```python
from build123d import *

# Parameters (mm, degrees)
F1_DEPTH     = 17.5
F2_T1_DEPTH  = 22.5
F3_T1_DEPTH  = 7
F3_T4_ANGLE  = 168.6544636073
F3_T6_ANGLE  = 168.6544636073
F3_T8_ANGLE  = 180
F3_T10_ANGLE = 168.6544636073
F3_T12_ANGLE = 168.6544636073
F3_T14_ANGLE = 180
F3_T16_ANGLE = 168.6544636073
F3_T18_ANGLE = 168.6544636073
F3_T20_ANGLE = 180
F3_T22_ANGLE = 168.6544636073
F3_T24_ANGLE = 168.6544636073
F3_T26_ANGLE = 180


# Not quite as in the source:
# - a fillet or chamfer that OpenCascade refuses, or shapes differently, is made with other operations: its cross-section is extruded or revolved along the edge and cut away or added


with BuildPart() as f1:
    # F0 (on Top) → F1 (new body)
    with BuildSketch(Plane.XY):
        with BuildLine():
            ThreePointArc((0, -2.75), (-2.75, 0), (0, 2.75))
            Line((0, 2.75), (8, 2.75))
            Line((8, 2.75), (8, 4.25))
            Line((8, 4.25), (0, 4.25))
            ThreePointArc((0, 4.25), (-4.25, 0), (0, -4.25))
            Line((0, -4.25), (8, -4.25))
            Line((8, -4.25), (8, -2.75))
            Line((8, -2.75), (0, -2.75))
        make_face()
    extrude(amount=F1_DEPTH)

    # F2: fillet of radius 1 on 4 edges, made by hand

    # F2_s2 → F2_t1 (cut)
    with BuildSketch(Plane.XY.offset(-2.5)):
        with BuildLine():
            ThreePointArc((8, -3.75), (7.7071067812, -3.0428932188), (7, -2.75))
            Line((7, -2.75), (8, -2.75))
            Line((8, -2.75), (8, -3.75))
        make_face()
        with BuildLine():
            ThreePointArc((7, -4.25), (7.7071067812, -3.9571067812), (8, -3.25))
            Line((8, -3.25), (8, -4.25))
            Line((8, -4.25), (7, -4.25))
        make_face()
        with BuildLine():
            ThreePointArc((7, 2.75), (7.7071067812, 3.0428932188), (8, 3.75))
            Line((8, 3.75), (8, 2.75))
            Line((8, 2.75), (7, 2.75))
        make_face()
        with BuildLine():
            ThreePointArc((8, 3.25), (7.7071067812, 3.9571067812), (7, 4.25))
            Line((7, 4.25), (8, 4.25))
            Line((8, 4.25), (8, 3.25))
        make_face()
    extrude(amount=F2_T1_DEPTH, mode=Mode.SUBTRACT)

    # F3: fillet of radius 0.65 on 20 edges, made by hand

    # F3_s2 → F3_t1 (cut)
    with BuildSketch(Plane.YZ):
        with BuildLine():
            ThreePointArc((-2.75, 0.65), (-2.9403805922, 0.1903805922), (-3.4, 0))
            Line((-3.4, 0), (-2.75, 0))
            Line((-2.75, 0), (-2.75, 0.65))
        make_face()
        with BuildLine():
            ThreePointArc((-3.6, 0), (-4.0596194078, 0.1903805922), (-4.25, 0.65))
            Line((-4.25, 0.65), (-4.25, 0))
            Line((-4.25, 0), (-3.6, 0))
        make_face()
        with BuildLine():
            ThreePointArc((3.6, 0), (4.0596194078, 0.1903805922), (4.25, 0.65))
            Line((4.25, 0.65), (4.25, 0))
            Line((4.25, 0), (3.6, 0))
        make_face()
        with BuildLine():
            ThreePointArc((2.75, 0.65), (2.9403805922, 0.1903805922), (3.4, 0))
            Line((3.4, 0), (2.75, 0))
            Line((2.75, 0), (2.75, 0.65))
        make_face()
        with BuildLine():
            ThreePointArc((-2.75, 16.85), (-2.9403805922, 17.3096194078), (-3.4, 17.5))
            Line((-3.4, 17.5), (-2.75, 17.5))
            Line((-2.75, 17.5), (-2.75, 16.85))
        make_face()
        with BuildLine():
            ThreePointArc((-3.6, 17.5), (-4.0596194078, 17.3096194078), (-4.25, 16.85))
            Line((-4.25, 16.85), (-4.25, 17.5))
            Line((-4.25, 17.5), (-3.6, 17.5))
        make_face()
        with BuildLine():
            ThreePointArc((3.6, 17.5), (4.0596194078, 17.3096194078), (4.25, 16.85))
            Line((4.25, 16.85), (4.25, 17.5))
            Line((4.25, 17.5), (3.6, 17.5))
        make_face()
        with BuildLine():
            ThreePointArc((2.75, 16.85), (2.9403805922, 17.3096194078), (3.4, 17.5))
            Line((3.4, 17.5), (2.75, 17.5))
            Line((2.75, 17.5), (2.75, 16.85))
        make_face()
    extrude(amount=F3_T1_DEPTH, mode=Mode.SUBTRACT)

    # F3_s3 → F3_t4 (revolve, cut)
    with BuildSketch(Plane.YZ.offset(7)):
        with BuildLine():
            ThreePointArc((-3.4, 0), (-2.9403805922, 0.1903805922), (-2.75, 0.65))
            Line((-2.75, 0.65), (-2.75, 0))
            Line((-2.75, 0), (-3.4, 0))
        make_face()
    revolve(axis=Axis((7, -3.75, 0), (0, 0, -1)), revolution_arc=F3_T4_ANGLE, mode=Mode.SUBTRACT)

    # F3_s5 → F3_t6 (revolve, cut)
    with BuildSketch(Plane(origin=(7.3559574547, -1.4759459573, 0), x_dir=(0, 0, 1), z_dir=(-0.9804586187, 0.1967254356, 0))):
        with BuildLine():
            ThreePointArc((0, -1.4594124616), (0.1903805922, -0.9997930538), (0.65, -0.8094124616))
            Line((0.65, -0.8094124616), (0, -0.8094124616))
            Line((0, -0.8094124616), (0, -1.4594124616))
        make_face()
    revolve(axis=Axis((7, -3.25, 0), (0, 0, -1)), revolution_arc=F3_T6_ANGLE, mode=Mode.SUBTRACT)

    # F3_s7 → F3_t8 (revolve, cut)
    with BuildSketch(Plane.YZ):
        with BuildLine():
            ThreePointArc((3.6, 0), (4.0596194078, 0.1903805922), (4.25, 0.65))
            Line((4.25, 0.65), (4.25, 0))
            Line((4.25, 0), (3.6, 0))
        make_face()
    revolve(axis=Axis((0, 0, 0), (0, 0, 1)), revolution_arc=F3_T8_ANGLE, mode=Mode.SUBTRACT)

    # F3_s9 → F3_t10 (revolve, cut)
    with BuildSketch(Plane.YZ.offset(7)):
        with BuildLine():
            ThreePointArc((3.6, 0), (4.0596194078, 0.1903805922), (4.25, 0.65))
            Line((4.25, 0.65), (4.25, 0))
            Line((4.25, 0), (3.6, 0))
        make_face()
    revolve(axis=Axis((7, 3.25, 0), (0, 0, -1)), revolution_arc=F3_T10_ANGLE, mode=Mode.SUBTRACT)

    # F3_s11 → F3_t12 (revolve, cut)
    with BuildSketch(Plane(origin=(6.0057894127, -1.2050396782, 0), x_dir=(0, 0, 1), z_dir=(-0.9804586187, 0.1967254356, 0))):
        with BuildLine():
            ThreePointArc((0, 5.4037978693), (0.1903805922, 5.8634172771), (0.65, 6.0537978693))
            Line((0.65, 6.0537978693), (0, 6.0537978693))
            Line((0, 6.0537978693), (0, 5.4037978693))
        make_face()
    revolve(axis=Axis((7, 3.75, 0), (0, 0, -1)), revolution_arc=F3_T12_ANGLE, mode=Mode.SUBTRACT)

    # F3_s13 → F3_t14 (revolve, cut)
    with BuildSketch(Plane.YZ):
        with BuildLine():
            ThreePointArc((-2.75, 0.65), (-2.9403805922, 0.1903805922), (-3.4, 0))
            Line((-3.4, 0), (-2.75, 0))
            Line((-2.75, 0), (-2.75, 0.65))
        make_face()
    revolve(axis=Axis((0, 0, 0), (0, 0, -1)), revolution_arc=F3_T14_ANGLE, mode=Mode.SUBTRACT)

    # F3_s15 → F3_t16 (revolve, cut)
    with BuildSketch(Plane.YZ.offset(7)):
        with BuildLine():
            ThreePointArc((-3.4, 17.5), (-2.9403805922, 17.3096194078), (-2.75, 16.85))
            Line((-2.75, 16.85), (-2.75, 17.5))
            Line((-2.75, 17.5), (-3.4, 17.5))
        make_face()
    revolve(axis=Axis((7, -3.75, 17.5), (0, 0, -1)), revolution_arc=F3_T16_ANGLE, mode=Mode.SUBTRACT)

    # F3_s17 → F3_t18 (revolve, cut)
    with BuildSketch(Plane(origin=(7.3559574547, -1.4759459573, 0), x_dir=(0, 0, 1), z_dir=(-0.9804586187, 0.1967254356, 0))):
        with BuildLine():
            ThreePointArc((17.5, -1.4594124616), (17.3096194078, -0.9997930538), (16.85, -0.8094124616))
            Line((16.85, -0.8094124616), (17.5, -0.8094124616))
            Line((17.5, -0.8094124616), (17.5, -1.4594124616))
        make_face()
    revolve(axis=Axis((7, -3.25, 17.5), (0, 0, -1)), revolution_arc=F3_T18_ANGLE, mode=Mode.SUBTRACT)

    # F3_s19 → F3_t20 (revolve, cut)
    with BuildSketch(Plane.YZ):
        with BuildLine():
            ThreePointArc((3.6, 17.5), (4.0596194078, 17.3096194078), (4.25, 16.85))
            Line((4.25, 16.85), (4.25, 17.5))
            Line((4.25, 17.5), (3.6, 17.5))
        make_face()
    revolve(axis=Axis((0, 0, 17.5), (0, 0, 1)), revolution_arc=F3_T20_ANGLE, mode=Mode.SUBTRACT)

    # F3_s21 → F3_t22 (revolve, cut)
    with BuildSketch(Plane.YZ.offset(7)):
        with BuildLine():
            ThreePointArc((3.6, 17.5), (4.0596194078, 17.3096194078), (4.25, 16.85))
            Line((4.25, 16.85), (4.25, 17.5))
            Line((4.25, 17.5), (3.6, 17.5))
        make_face()
    revolve(axis=Axis((7, 3.25, 17.5), (0, 0, -1)), revolution_arc=F3_T22_ANGLE, mode=Mode.SUBTRACT)

    # F3_s23 → F3_t24 (revolve, cut)
    with BuildSketch(Plane(origin=(6.0057894127, -1.2050396782, 0), x_dir=(0, 0, 1), z_dir=(-0.9804586187, 0.1967254356, 0))):
        with BuildLine():
            ThreePointArc((17.5, 5.4037978693), (17.3096194078, 5.8634172771), (16.85, 6.0537978693))
            Line((16.85, 6.0537978693), (17.5, 6.0537978693))
            Line((17.5, 6.0537978693), (17.5, 5.4037978693))
        make_face()
    revolve(axis=Axis((7, 3.75, 17.5), (0, 0, -1)), revolution_arc=F3_T24_ANGLE, mode=Mode.SUBTRACT)

    # F3_s25 → F3_t26 (revolve, cut)
    with BuildSketch(Plane.YZ):
        with BuildLine():
            ThreePointArc((-2.75, 16.85), (-2.9403805922, 17.3096194078), (-3.4, 17.5))
            Line((-3.4, 17.5), (-2.75, 17.5))
            Line((-2.75, 17.5), (-2.75, 16.85))
        make_face()
    revolve(axis=Axis((0, 0, 17.5), (0, 0, -1)), revolution_arc=F3_T26_ANGLE, mode=Mode.SUBTRACT)


solid = f1.part
```
Geometry check sheet. Reference: the model listing, model coordinates, mm. A direction names the side the tool comes from. Coordinates: 2 decimals unless noted, no trailing zeros. Loops run counter-clockwise (first coordinate to the right, second up) from the corner with the lowest first, then second, coordinate; pieces in that order, holes last.
Item 1: Sectioned sample at B-B, the plane y = 0. Record the boundary of the cut face in (x, z).
Item 2: Sectioned sample at A-A, the plane x = 6.75. Record the boundary of the cut face in (y, z), then the cut area to 3 significant figures.
Item 3: Go/stop test with flat-tipped pins: pin 1 Ø5 at (y, z) = (0, 11) entering from +X; pin 2 Ø1.5 at (x, z) = (-2, 5) entering from -Y; pin 3 Ø1.5 at (x, z) = (-1, 10.5) entering from +Y; pin 4 Ø2 at (x, y) = (3.5, 1) entering from +Z. Record where each tip stops, or that it passes through.
Item 4: Thickness scan on line 1 (Y direction, x = 5.5, z = 5.75); line 2 (Y direction, x = -1.75, z = 9.5); line 3 (Z direction, x = -2, y = -3.5). Record the ranges inside material, lowest first.
Item 5: Access from +Z, -Z, +X, -X, +Y, -Y to the whole of each face (thin tool, end or side, straight path). Record for faces 1 (the face through (7.62, -2.965, 8.637)), 2 (the face through (7.605, -4.046, 8.637)).
Item 6: Sectioned sample at C-C, the plane z = 2.25. Record the boundary of the cut face in (x, y), then the cut area to 3 significant figures.
Item 7: Release check for a two-part mould opening along Y. For faces 3 (the face through (-2.75, -0.06, 8.64)), 4 (the face through (4, 4.25, 9)), 5 (the face through (3, -4.25, 9)), 6 (the face through (-4.25, 0.09, 8.64)) record: released by +Y, released by -Y, zero draft, split by the parting line, or undercut.
Check result:
1. outline: (-4.25, 0.65) arc R0.65 ccw to (-3.6, 0) - (-3.4, 0) arc R0.65 ccw to (-2.75, 0.65) - (-2.75, 16.85) arc R0.65 ccw to (-3.4, 17.5) - (-3.6, 17.5) arc R0.65 ccw to (-4.25, 16.85) - close
2. outline: (-4.25, 0.65) arc R0.65 ccw to (-3.6, 0) - (-3.4, 0) arc R0.65 ccw to (-2.75, 0.65) - (-2.75, 16.85) arc R0.65 ccw to (-3.4, 17.5) - (-3.6, 17.5) arc R0.65 ccw to (-4.25, 16.85) - close; (2.75, 0.65) arc R0.65 ccw to (3.4, 0) - (3.6, 0) arc R0.65 ccw to (4.25, 0.65) - (4.25, 16.85) arc R0.65 ccw to (3.6, 17.5) - (3.4, 17.5) arc R0.65 ccw to (2.75, 16.85) - close
2. area: 51.8 mm2
3. pin 1: stops at x = -1.15
3. pin 2: stops at y = -4.06
3. pin 3: stops at y = 4.24
3. pin 4: passes through
4. line 1: y = -4.25 to -2.75, 2.75 to 4.25
4. line 2: y = -3.87 to -2.12, 2.12 to 3.87
4. line 3: z = 0.16 to 17.34
5. face 1: +Z, -Z, +X
5. face 2: +Z, -Z, +X, -Y
6. outline: (0, -4.25) - (7, -4.25) arc R1 ccw to (7.97, -3.5) arc R1 ccw to (7, -2.75) - (0, -2.75) arc R2.75 cw to (0, 2.75) - (7, 2.75) arc R1 ccw to (7.97, 3.5) arc R1 ccw to (7, 4.25) - (0, 4.25) arc R4.25 ccw to start
6. area: 39.6 mm2
7. face 3: undercut
7. face 4: released by +Y
7. face 5: released by -Y
7. face 6: split by the parting line
